Read the model definition and answer for the solid it produces. Units are mm, in the model's axes. Face numbers are marked on the shaded views. A direction names the side the tool comes from. Round coordinates to 2 decimals unless told otherwise and drop trailing zeros. Write each loop counter-clockwise with the first axis right and the second up, starting at its lowest first coordinate (ties: lowest second). Pieces come first, ordered by that corner, then holes. Notation, with made-up numbers: (-6, -32.75) -> (47, -32.75) arc R25 cw to (47, -14.75) -> close; hole circle Ø10 at (-28, 20.5). An arc over 180 degrees is marked (long way). Return JSON: item names as keys, results as strings. Group by question number.
(1) A cutting plane is placed at C-C on y = -50.8. Give the vertices of the cut face in (x, z), then the cut area to 3 significant figures.
(2) A cutting plane is placed at A-A on z = 31.75. Give the vertices of the cut face in (x, y).
(3) A cutting plane is placed at B-B on x = 0. Give the vertices of the cut face in (y, z).
(4) Straight lines are drawn through the part: line 1 (X direction, y = 50, z = 5); line 2 (Y direction, x = -76.2, z = 6); line 3 (X direction, y = 51, z = 16). For each, find the intervals that lie inside material, in ascending order.
(5) The mould has two halves that part along X. Classify the marked faces 1, 2 and 3: released by +X, released by -X, zero draft, split by the parting line, or undercut.
(6) For the marked faces 4, 5, 6, 7 and 8, determine the directions among +Z, -Z, +X, -X, +Y, -Y from which every point of the face is accessible in a straight line to the end or side of a thin tool.
(7) A cutting plane is placed at D-D on z = 7. Give the vertices of the cut face in (x, y), then the cut area to 3 significant figures.
(8) Given pin 1 (9.5 mm diameter, centred on x = 112, z = 29.5, fed in from +Y); pin 2 (21 mm diameter, centred on x = -74.5, z = 7, fed in from -Y); pin 3 (12.5 mm diameter, centred on x = 10.5, z = 27.5, fed in from +Y), each flat-ended and moving along its own axis, determine where each tip first touches the part or whether it passes through.
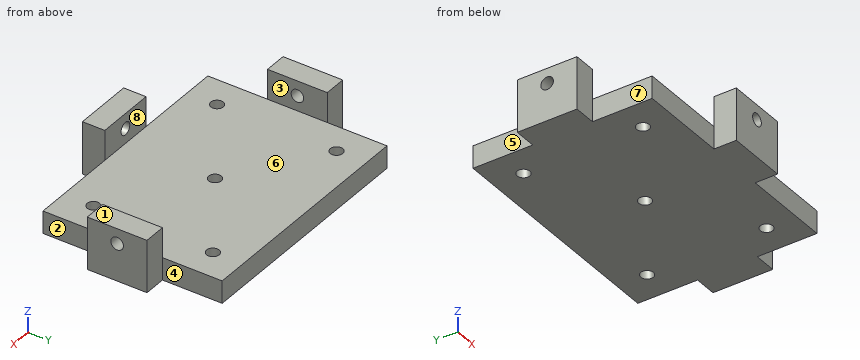
```python
from build123d import *

# Parameters (mm, degrees)
F0_W     = 203.2
F0_H     = 152.4
F1_DEPTH = 19.05
F3_D     = 10.71626
F4_W     = 19.05
F4_H     = 50.8
F4_W_2   = 50.8
F4_H_2   = 19.05
F5_DEPTH = 44.45
F7_D     = 10.71626
F9_D     = 10.71626


with BuildPart() as f1:
    # F0 (on Top) → F1 (new body)
    with BuildSketch(Plane.XY):
        Rectangle(F0_W, F0_H)
    extrude(amount=F1_DEPTH)

    # F3 (through all)
    with Locations(Plane.XY.offset(19.05)):
        with Locations((-76.2, 50.8), (76.2, 50.8), (0, 0), (-76.2, -50.8), (76.2, -50.8)):
            Hole(F3_D / 2)

    # F4 (on face) → F5 (join)
    with BuildSketch(Plane.XY):
        with Locations((-111.125, 0)):
            Rectangle(F4_W, F4_H)
        with Locations((0, -85.725)):
            Rectangle(F4_W_2, F4_H_2)
        with Locations((111.125, 0)):
            Rectangle(F4_W, F4_H)
    extrude(amount=F5_DEPTH)

    # F7 (through all)
    with Locations(Plane.XZ.offset(95.25)):
        with Locations((0, 31.75)):
            Hole(F7_D / 2)

    # F9 (through all)
    with Locations(Plane(origin=(-120.65, 0, 0), x_dir=(0, -1, 0), z_dir=(-1, 0, 0))):
        with Locations((0, 31.75)):
            Hole(F9_D / 2)


solid = f1.part
```
Checks:
{
 "1": {"outline": "(-101.6, 0) -> (-81.56, 0) -> (-81.56, 19.05) -> (-101.6, 19.05) -> close; (-70.84, 0) -> (70.84, 0) -> (70.84, 19.05) -> (-70.84, 19.05) -> close; (81.56, 0) -> (101.6, 0) -> (101.6, 19.05) -> (81.56, 19.05) -> close", "area": "3,460 mm^2"},
 "2": {"outline": "(-120.65, -25.4) -> (-101.6, -25.4) -> (-101.6, -5.36) -> (-120.65, -5.36) -> close; (-120.65, 5.36) -> (-101.6, 5.36) -> (-101.6, 25.4) -> (-120.65, 25.4) -> close; (-25.4, -95.25) -> (-5.36, -95.25) -> (-5.36, -76.2) -> (-25.4, -76.2) -> close; (5.36, -95.25) -> (25.4, -95.25) -> (25.4, -76.2) -> (5.36, -76.2) -> close; (101.6, -25.4) -> (120.65, -25.4) -> (120.65, -5.36) -> (101.6, -5.36) -> close; (101.6, 5.36) -> (120.65, 5.36) -> (120.65, 25.4) -> (101.6, 25.4) -> close"},
 "3": {"outline": "(-95.25, 0) -> (-5.36, 0) -> (-5.36, 19.05) -> (-76.2, 19.05) -> (-76.2, 26.39) -> (-95.25, 26.39) -> close; (-95.25, 37.11) -> (-76.2, 37.11) -> (-76.2, 44.45) -> (-95.25, 44.45) -> close; (5.36, 0) -> (76.2, 0) -> (76.2, 19.05) -> (5.36, 19.05) -> close"},
 "4": {"line 1": "x = -101.6 to -81.5, -70.9 to 70.9, 81.5 to 101.6", "line 2": "y = -76.2 to -56.16, -45.44 to 45.44, 56.16 to 76.2", "line 3": "x = -101.6 to -81.55, -70.85 to 70.85, 81.55 to 101.6"},
 "5": {"face 1": "zero draft", "face 2": "released by +X", "face 3": "undercut"},
 "6": {"face 4": "+Z, -Z, +X, +Y", "face 5": "+Z, -Z, -X, +Y", "face 6": "+Z, +Y", "face 7": "+Z, -Z, -X, -Y", "face 8": "+Z, +X, -X, +Y"},
 "7": {"outline": "(-120.65, -25.4) -> (-101.6, -25.4) -> (-101.6, -76.2) -> (-25.4, -76.2) -> (-25.4, -95.25) -> (25.4, -95.25) -> (25.4, -76.2) -> (101.6, -76.2) -> (101.6, -25.4) -> (120.65, -25.4) -> (120.65, 25.4) -> (101.6, 25.4) -> (101.6, 76.2) -> (-101.6, 76.2) -> (-101.6, 25.4) -> (-120.65, 25.4) -> close; hole circle Ø10.72 at (-76.2, -50.8); hole circle Ø10.72 at (-76.2, 50.8); hole circle Ø10.72 at (0, 0); hole circle Ø10.72 at (76.2, -50.8); hole circle Ø10.72 at (76.2, 50.8)", "area": "33,400 mm^2"},
 "8": {"pin 1": "stops at y = 25.4", "pin 2": "stops at y = -76.2", "pin 3": "stops at y = -76.2"}
}
